Here's how the part is built. I have some questions about the finished solid (model axes, mm). A direction names the side the tool comes from. Coordinates: 2 decimals unless noted, no trailing zeros. Write each loop counter-clockwise with the first axis right and the second up, starting at its lowest first coordinate (ties: lowest second). Pieces come first, ordered by that corner, then holes. Notation, with made-up numbers: (13, -28.5) - (40, -28.5) arc R19 ccw to (40, 5.5) - close; hole circle Ø2 at (29.25, 53.25). An arc over 180 degrees is marked (long way). Answer in a Markdown table with one row per item. Add a question column.
Item 1: Imagine slicing it at A-A (x = 77.5). Please give me the cut outline in (y, z).
Item 2: I'm going to push flat-ended pins straight in: pin 1 (5 mm diameter, centred on x = 80, y = -35.5, fed in from +Z); pin 2 (19 mm diameter, centred on x = 63.5, y = -76.5, fed in from -Z); pin 3 (4 mm diameter, centred on x = 34, y = -44.5, fed in from -Z). Where does each tip first touch, or does it pass through?
Item 3: Imagine slicing it at B-B (z = -33.5). Please give me the cut outline in (x, y).
Item 4: If I drill on probe 1 along Z at (x, y) = (74, -68); probe 2 along X at (y, z) = (-18, 3); probe 3 along X at (y, z) = (-8.5, -49), over which ranges is the centre line in solid material (lowest first)? Write a range as from..to.
Item 5: Imagine slicing it at D-D (y = -35). Please give me the cut outline in (x, z).
Item 6: Which directions (+Z, -Z, +X, -X, +Y, -Y) give clear straight access to the entire face, cutting with the end or side of a thin tool? Please do faces 4 (the face through (23, -63, -28.301)), 5 (the face through (29.455, -63, -45)), 6 (the face through (118.381, -86, 81)).
Item 7: Imagine slicing it at C-C (y = -92.5). Please give me the cut outline in (x, z), plus the area to 3 significant figures.
Item 8: We'd pull the mould along Z, two halves only. Please class faces 1 (the face through (49, -22.86, 99)), 2 (the face through (48, -63, 9.799)), 3 (the face through (2, -63, -61.448)): +Z half, -Z half, draft (parallel to the pull), parting line (faces both ways), or undercut.
from build123d import *

# Parameters (mm, degrees)
BOSS_EXTRUDE1_DEPTH = 127
SKETCH2_W           = 139.7
SKETCH2_H           = 83.185
BOSS_EXTRUDE2_DEPTH = 83.82
SKETCH3_R           = 24.13
BOSS_EXTRUDE3_DEPTH = 20.32


with BuildPart() as part:
    # Sketch1 → Boss-Extrude1 (new body)
    with BuildSketch(Plane(origin=(0, 0, 0), x_dir=(1, 0, 0), z_dir=(0, 1, 0))):
        Polygon((16.729923946, 28.301454676), (16.729923946, -9.798545324), (80.331523946, -9.798545324), (80.331523946, 28.301454676), (67.606123946, 28.301454676), (67.606123946, 61.448454676), (122.393923946, 61.448454676), (122.393923946, -40.278545324), (-25.332476054, -40.278545324), (-25.332476054, 61.448454676), (29.455323946, 61.448454676), (29.455323946, 28.301454676), align=None)
    extrude(amount=-BOSS_EXTRUDE1_DEPTH)

    # Sketch2 → Boss-Extrude2 (add)
    with BuildSketch(Plane.XZ.offset(127)):
        with Locations((48.530723946, 81.871045324)):
            Rectangle(SKETCH2_W, SKETCH2_H)
    extrude(amount=-BOSS_EXTRUDE2_DEPTH)

    # Sketch3 → Boss-Extrude3 (add)
    with BuildSketch(Plane(origin=(0, -43.18, 0), x_dir=(1, 0, 0), z_dir=(0, 1, 0))):
        with Locations(Location((48.530723946, -99.333545324, 0), (0, 0, 270))):
            Circle(SKETCH3_R)
    extrude(amount=BOSS_EXTRUDE3_DEPTH)


solid = part.part
Here are the results:
| question | item | result |
|---|---|---|
| 1 | outline | (-127, -61.45) - (0, -61.45) - (0, -28.3) - (-127, -28.3) - close; (-127, 9.8) - (0, 9.8) - (0, 40.28) - (-43.18, 40.28) - (-43.18, 123.46) - (-127, 123.46) - close |
| 2 | pin 1 | stops at z = 40.28 |
| 2 | pin 2 | stops at z = -61.45 |
| 2 | pin 3 | stops at z = 9.8 |
| 3 | outline | (-25.33, -127) - (29.46, -127) - (29.46, 0) - (-25.33, 0) - close; (67.61, -127) - (122.39, -127) - (122.39, 0) - (67.61, 0) - close |
| 4 | probe 1 | z = -61.45..-28.3, 9.8..123.46 |
| 4 | probe 2 | x = -25.33..16.73, 80.33..122.39 |
| 4 | probe 3 | x = -25.33..29.46, 67.61..122.39 |
| 5 | outline | (-25.33, -61.45) - (29.46, -61.45) - (29.46, -28.3) - (16.73, -28.3) - (16.73, 9.8) - (80.33, 9.8) - (80.33, -28.3) - (67.61, -28.3) - (67.61, -61.45) - (122.39, -61.45) - (122.39, 40.28) - (-25.33, 40.28) - close; circle Ø48.26 at (48.53, 99.33) |
| 6 | face 4 | +Y, -Y |
| 6 | face 5 | -Z, +Y, -Y |
| 6 | face 6 | +Z, +X, +Y, -Y |
| 7 | outline | (-25.33, -61.45) - (29.46, -61.45) - (29.46, -28.3) - (16.73, -28.3) - (16.73, 9.8) - (80.33, 9.8) - (80.33, -28.3) - (67.61, -28.3) - (67.61, -61.45) - (122.39, -61.45) - (122.39, 40.28) - (118.38, 40.28) - (118.38, 123.46) - (-21.32, 123.46) - (-21.32, 40.28) - (-25.33, 40.28) - close |
| 7 | area | 23,000 mm2 |
| 8 | face 1 | draft |
| 8 | face 2 | undercut |
| 8 | face 3 | -Z half |
